Part print with two shaded views. Sizes in mm from the minimum x, y, z corner. A direction names the side the tool comes from. Give positions to 0.01 mm unless a question says otherwise; leave off trailing zeros. Write each loop counter-clockwise with the first axis right and the second up, starting at its lowest first coordinate (ties: lowest second). Pieces come first, ordered by that corner, then holes. Notation, with made-up numbers: (-15.5, 33) - (11.5, 33) arc R31 cw to (11.5, 60) - close; hole circle Ø2 at (4, 77). An arc over 180 degrees is marked (long way). One line per item, written item: value. Start each with the question number.
(1) Cut at B-B, the plane y = 1.6. List the corners of the cut face in (x, z).
(2) 3-axis set-ups, long thin cutter, end or side, ignore diameter. For the marked faces 1, 2 and 3: which of +Z, -Z, +X, -X, +Y, -Y reach the whole face in a straight line?
(3) Cut at A-A, the plane z = 0.4. List the corners of the cut face in (x, y), and give its area (3 significant figures).
(4) Probe L1, parallel to X at y = 1.3, z = 0.7; L2, parallel to Y at x = 1.05, z = 0.2; L3, parallel to X at y = 0.65, z = 0.2. List the from-to ranges inside material, lowest first.
(5) Cut at C-C, the plane x = 4.9. List the corners of the cut face in (y, z).
(6) Drop a flat-ended pin along its axis: P1, Ø0.5, axis at y = 2.5, z = 0.5, coming from the -X side. Give the stop position or say it passes through.
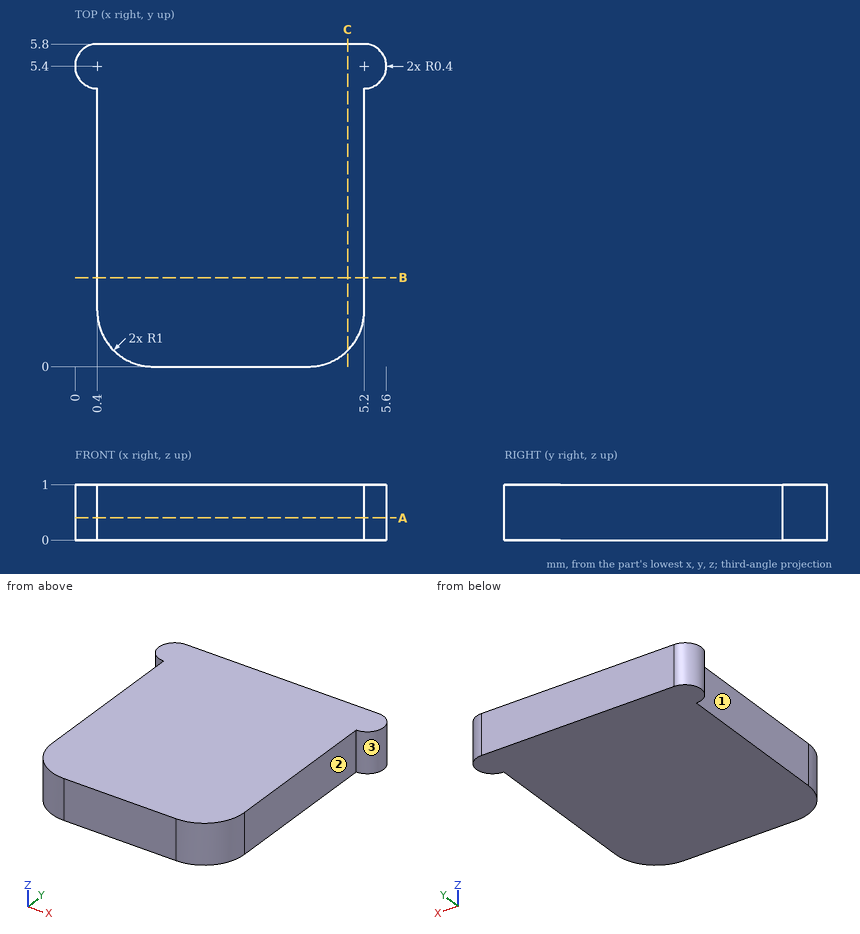
Answers follow:
1. outline: (0.4, 0) - (5.2, 0) - (5.2, 1) - (0.4, 1) - close
2. face 1: +Z, -Z, -X, -Y
2. face 2: +Z, -Z, +X, -Y
2. face 3: +Z, -Z, +X
3. outline: (0.4, 1) arc R1 ccw to (1.4, 0) - (4.2, 0) arc R1 ccw to (5.2, 1) - (5.2, 5) arc R0.4 ccw to (5.2, 5.8) - (0.4, 5.8) arc R0.4 ccw to (0.4, 5) - close
3. area: 27.9 mm²
4. L1: x = 0.4 to 5.2
4. L2: y = 0.06 to 5.8
4. L3: x = 0.46 to 5.14
5. outline: (0.29, 0) - (5.8, 0) - (5.8, 1) - (0.29, 1) - close
6. P1: stops at x = 0.4
